Input: part model. Units: mm. Frame: model coordinates. A direction names the side the tool comes from. Coordinates: 2 decimals unless noted, no trailing zeros. Order: outer loops, then holes, each group sorted by start corner. A loop starts at its lowest first (then second) coordinate and runs counter-clockwise, first axis right, second up.
from build123d import *

# Parameters (mm, degrees)
SKETCH1_W            = 2.5
SKETCH1_H            = 10
BOSS_EXTRUDE1_DEPTH  = 1.52
SKETCH2_W            = 0.8
SKETCH2_H            = 0.8
CUT_EXTRUDE1_DEPTH   = 7
CHAMFER_1_SIZE       = 0.4
BOSS_EXTRUDE2_DEPTH  = 0.2
MIRROR_START         = -1.52
MIRROR_1_DEPTH       = 3.04
MIRROR_1_2_DEPTH     = 0.72
MIRROR_START_2       = 0.8
MIRROR_1_3_DEPTH     = 0.72
MIRROR_START_3       = -0.124264069
MIRROR_1_4_OUTLINE_W = 0.4
MIRROR_1_4_OUTLINE_H = 2.2
MIRROR_1_4_DEPTH     = 0.248528138
MIRROR_START_4       = 1
MIRROR_1_5_DEPTH     = 2.32
MIRROR_START_5       = 2.34
MIRROR_1_6_DEPTH     = 0.4
LPATTERN1_COUNT      = 3
LPATTERN1_PITCH      = 2.54


with BuildPart() as part:
    # Sketch1 → Boss-Extrude1 (new, symmetric)
    with BuildSketch(Plane(origin=(0, 0, 0), x_dir=(0, -1, 0), z_dir=(1, 0, 0))):
        with Locations((-0.02, -5)):
            Rectangle(SKETCH1_W, SKETCH1_H)
    extrude(amount=BOSS_EXTRUDE1_DEPTH, both=True)

    # Sketch2 → Cut-Extrude1 (cut)
    with BuildSketch(Plane(origin=(0, 0, 10), x_dir=(-1, 0, 0), z_dir=(0, 0, 1))):
        with Locations((0, -0.02)):
            Rectangle(SKETCH2_W, SKETCH2_H)
    extrude(amount=-CUT_EXTRUDE1_DEPTH, mode=Mode.SUBTRACT)

    # Фаска1
    chamfer_1_edges = [part.edges().sort_by_distance(p)[0] for p in [
        (-0.4, 0.02, 10),
        (0, -0.38, 10),
        (0.4, 0.02, 10),
        (0, 0.42, 10),
    ]]
    chamfer(chamfer_1_edges, length=CHAMFER_1_SIZE)

    # Sketch3 → Boss-Extrude2 (add, symmetric)
    with BuildSketch(Plane(origin=(0, 0, 0), x_dir=(1, 0, 0), z_dir=(0, 1, 0))):
        Polygon((-0.3, 0), (-0.3, 2.024264069), (-0.124264069, 2.2), (0.124264069, 2.2), (0.3, 2.024264069), (0.3, 0), align=None)
    extrude(amount=BOSS_EXTRUDE2_DEPTH, both=True)

    # Зеркальное отражение1: read off the stored shape, not the designer's step
    # Зеркальное отражение1 outline → Зеркальное отражение1 (add)
    with BuildSketch(Plane.YZ.offset(MIRROR_START)):
        Polygon((1.72, 10), (1.27, 10), (1.27, 0), (3.77, 0), (3.77, 10), (3.32, 10), (2.92, 9.6), (2.92, 3), (2.12, 3), (2.12, 9.6), align=None)
    extrude(amount=MIRROR_1_DEPTH)

    # Mirror 1 2 outline → Mirror 1 2 (add)
    with BuildSketch(Plane.YZ.offset(MIRROR_START)):
        Polygon((3.32, 10), (1.72, 10), (2.12, 9.6), (2.12, 3), (2.92, 3), (2.92, 9.6), align=None)
    extrude(amount=MIRROR_1_2_DEPTH)

    # Mirror 1 3 outline → Mirror 1 3 (add)
    with BuildSketch(Plane.YZ.offset(MIRROR_START_2)):
        Polygon((3.32, 10), (1.72, 10), (2.12, 9.6), (2.12, 3), (2.92, 3), (2.92, 9.6), align=None)
    extrude(amount=MIRROR_1_3_DEPTH)

    # Mirror 1 4 outline → Mirror 1 4 (add)
    with BuildSketch(Plane.YZ.offset(MIRROR_START_3)):
        with Locations((2.54, -1.1)):
            Rectangle(MIRROR_1_4_OUTLINE_W, MIRROR_1_4_OUTLINE_H)
    extrude(amount=MIRROR_1_4_DEPTH)

    # Mirror 1 5 outline → Mirror 1 5 (add)
    with BuildSketch(Plane(origin=(0, 0, 0), x_dir=(1, 0, 0), z_dir=(0, 1, 0)).offset(MIRROR_START_4)):
        Polygon((-0.8, -10), (-0.4, -9.6), (-0.4, -3), (-0.8, -3), align=None)
        Polygon((0.8, -3), (0.4, -3), (0.4, -9.6), (0.8, -10), align=None)
    extrude(amount=MIRROR_1_5_DEPTH)

    # Mirror 1 6 outline → Mirror 1 6 (add)
    with BuildSketch(Plane(origin=(0, 0, 0), x_dir=(1, 0, 0), z_dir=(0, 1, 0)).offset(MIRROR_START_5)):
        Polygon((0.124264069, 0), (0.3, 0), (0.3, 2.024264069), (0.124264069, 2.2), align=None)
        Polygon((-0.3, 0), (-0.124264069, 0), (-0.124264069, 2.2), (-0.3, 2.024264069), align=None)
    extrude(amount=MIRROR_1_6_DEPTH)


with BuildPart() as lpattern1_1:
    # LPattern1: pattern copy
    add(part.part.moved(Location(Vector(1, 0, 0) * (1 * LPATTERN1_PITCH))))


with BuildPart() as lpattern1_2:
    # LPattern1: pattern copy
    add(part.part.moved(Location(Vector(1, 0, 0) * (2 * LPATTERN1_PITCH))))

    # Combine 1: union LPattern1_1, part
    add(lpattern1_1.part)
    add(part.part)


solid = lpattern1_2.part
Item 1: Cut plane C-C on x = 1. Return loops of the section in (y, z), then the cut area to 3 significant figures.
Response values:
outline: (-1.23, 0) - (3.77, 0) - (3.77, 10) - (-1.23, 10) - close
area: 50.0 mm2
Item 2: Cut plane B-B on y = 1.3. Return loops of the section in (x, z).
Response values:
outline: (-1.52, 0) - (6.6, 0) - (6.6, 10) - (-1.52, 10) - close
Item 3: Ray query, probe 1 along X at (y, z) = (2.65, 5.75); probe 2 along Y at (x, z) = (0, 5.5); probe 3 along Z at (x, y) = (1.5, 3.15). Return the intervals inside material, ascending.
Response values:
probe 1: x = -1.52 to -0.4, 0.4 to 2.14, 2.94 to 4.68, 5.48 to 6.6
probe 2: y = -1.23 to -0.38, 0.42 to 2.12, 2.92 to 3.77
probe 3: z = 0 to 10
Item 4: Pin query (flat end, axial travel): pin 1 Ø0.9 at (x, y) = (0, 0) entering from +Z; pin 2 Ø0.5 at (x, z) = (0, -1.5) entering from -Y; pin 3 Ø1.5 at (x, y) = (4, 2.5) entering from -Z. Return the tip coordinate at first contact, or that it passes through.
Response values:
pin 1: stops at z = 9.67
pin 2: stops at y = -0.2
pin 3: stops at z = 0
Item 5: Cut plane A-A on z = 3.25. Return loops of the section in (x, y), then the cut area to 3 significant figures.
Response values:
outline: (-1.52, -1.23) - (6.6, -1.23) - (6.6, 3.77) - (-1.52, 3.77) - close; hole (-0.4, -0.38) - (0.4, -0.38) - (0.4, 0.42) - (-0.4, 0.42) - close; hole (-0.4, 2.12) - (0.4, 2.12) - (0.4, 2.92) - (-0.4, 2.92) - close; hole (2.14, -0.38) - (2.94, -0.38) - (2.94, 0.42) - (2.14, 0.42) - close; hole (2.14, 2.12) - (2.94, 2.12) - (2.94, 2.92) - (2.14, 2.92) - close; hole (4.68, -0.38) - (5.48, -0.38) - (5.48, 0.42) - (4.68, 0.42) - close; hole (4.68, 2.12) - (5.48, 2.12) - (5.48, 2.92) - (4.68, 2.92) - close
area: 36.8 mm2
Item 6: Access query for faces 1 (the face through (6.6, 1, 5)), 2 (the face through (2.5, 0.42, 6.3)). Directions: +Z, -Z, +X, -X, +Y, -Y. A direction counts if a zero-diameter tool reaches every point of the face in a straight line with its end or side. Return the directions, or none.
Response values:
face 1: +Z, -Z, +X, +Y, -Y
face 2: +Z
Item 7: Draft query along Y for faces 3 (the face through (2, 3.77, 5)), 4 (the face through (5, 2.92, 6)), 5 (the face through (5, -0.38, 6)), 6 (the face through (-1.52, 1, 5)). Return one class per face: pulls with the +Y half, pulls with the -Y half, needs draft (parallel to the pull), parting line crosses it, or undercut.
Response values:
face 3: pulls with the +Y half
face 4: undercut
face 5: undercut
face 6: needs draft
